Verification items for the finished model (mm, model axes). A direction names the side the tool comes from. Round coordinates to 2 decimals unless told otherwise and drop trailing zeros. Order: outer loops, then holes, each group sorted by start corner. A loop starts at its lowest first (then second) coordinate and runs counter-clockwise, first axis right, second up. Notation, with made-up numbers: M 84,73 L 130,73 A24 ccw 130,92 Z; hole C 27,73 d7. An arc over 180 degrees is marked long. Answer as a JSON object with one key per item and string values. Group by question number.
```python
from build123d import *

# Parameters (mm, degrees)
F_8_CLEARANCE_HOLE1_D     = 4.4958
F_8_CLEARANCE_HOLE1_DEPTH = 3.176
CIRPATTERN1_COUNT         = 6
SKETCH4_R                 = 63.5
CUT_EXTRUDE1_DEPTH        = 13.7


with BuildPart() as part:
    # Sketch1 → Revolve1 (revolve)
    with BuildSketch(Plane(origin=(0, 0, 0), x_dir=(0, 0, -1), z_dir=(1, 0, 0))):
        Polygon((66.675, 0), (69.85, 0), (69.85, 9.525), (82.55, 9.525), (82.55, 12.7), (0, 12.7), (0, 9.525), (66.675, 9.525), align=None)
    revolve(axis=Axis((0, 0, 0), (0, 1, 0)))

    # #8 Clearance Hole1
    with Locations(Plane(origin=(0, 12.7, 0), x_dir=(1, 0, 0), z_dir=(0, 1, 0))):
        with Locations((0, 76.2)):
            f_8_clearance_hole1 = Hole(F_8_CLEARANCE_HOLE1_D / 2, depth=F_8_CLEARANCE_HOLE1_DEPTH)

    # CirPattern1: #8 Clearance Hole1 ×6 about axis
    cirpattern1_axis = Axis((0, 0, 0), (0, 1, 0))
    for i in range(1, CIRPATTERN1_COUNT):
        add(f_8_clearance_hole1.rotate(cirpattern1_axis, i * 360 / CIRPATTERN1_COUNT), mode=Mode.SUBTRACT)

    # Sketch4 → Cut-Extrude1 (cut, through all)
    with BuildSketch(Plane(origin=(0, 12.7, 0), x_dir=(1, 0, 0), z_dir=(0, 1, 0))):
        Circle(SKETCH4_R)
    extrude(amount=-CUT_EXTRUDE1_DEPTH, mode=Mode.SUBTRACT)


solid = part.part
```
Q1. Cross-section at D-D, the plane x = -32. Record the cut outline in (y, z) (3 decimals).
Q2. Gauge pin test, flat ends, axial feed: pin 1 Ø7 at (x, z) = (0, 76.2) entering from -Y (3 decimals); pin 2 Ø4 at (x, y) = (-21, 10.5) entering from -Z; pin 3 Ø3.5 at (x, z) = (-65.99, 38.1) entering from +Y; pin 4 Ø1 at (y, z) = (9.5, -34) entering from -X. Record the tip position at first contact, or that the pin passes through.
Q3. Tool access check on faces 4 (the face through (26, 0, 62)), 5 (the face through (-20.027, 4.696, -63.596)). Record the directions out of +Z, -Z, +X, -X, +Y, -Y that give a thin tool (end or side, any length) a straight path to the whole face; none if there is none.
Q4. Cross-section at A-A, the plane z = 0. Record the cut outline in (x, y) (3 decimals).
Q5. Thickness scan on line 1 (Z direction, x = 0, y = 12); line 2 (X direction, y = 11.2, z = -38.1); line 3 (X direction, y = 11.6, z = 0). Record the ranges inside material, lowest first. Write a range as from..to.
Q6. Release check for a two-part mould opening along X. For faces 1 (the face through (42.503, 4.829, 55.431)), 2 (the face through (-0.29, 11.09, 78.43)), 3 (the face through (-19, 9.525, -68)) record: released by +X, released by -X, zero draft, split by the parting line, or undercut.
Q7. Cross-section at C-C, the plane z = 38.1. Record the cut outline in (x, y) (3 decimals), then the cut area to 3 significant figures.
Q8. Cross-section at B-B, the plane x = 0. Record the cut outline in (y, z) (3 decimals).
Conclusion:
{
 "1": {"outline": "M 0,-62.089 L 9.525,-62.089 L 9.525,-76.095 L 12.7,-76.095 L 12.7,-54.848 L 9.525,-54.848 L 9.525,-58.494 L 0,-58.494 Z; M 0,58.494 L 9.525,58.494 L 9.525,54.848 L 12.7,54.848 L 12.7,76.095 L 9.525,76.095 L 9.525,62.089 L 0,62.089 Z"},
 "2": {"pin 1": "y = 9.525", "pin 2": "z = -80.33", "pin 3": "through", "pin 4": "x = -75.45"},
 "3": {"face 4": "+Z, -Z, +X, -X, -Y", "face 5": "-Y"},
 "4": {"outline": "M -82.55,9.525 L -69.85,9.525 L -69.85,0 L -66.675,0 L -66.675,9.525 L -63.5,9.525 L -63.5,12.7 L -82.55,12.7 Z; M 63.5,9.525 L 66.675,9.525 L 66.675,0 L 69.85,0 L 69.85,9.525 L 82.55,9.525 L 82.55,12.7 L 63.5,12.7 Z"},
 "5": {"line 1": "-82.55..-78.45, -73.95..-63.5, 63.5..73.95, 78.45..82.55", "line 2": "-73.23..-68.24, -63.74..-50.8, 50.8..63.74, 68.24..73.23", "line 3": "-82.55..-63.5, 63.5..82.55"},
 "6": {"face 1": "split by the parting line", "face 2": "undercut", "face 3": "zero draft"},
 "7": {"outline": "M -73.232,9.525 L -68.239,9.525 L -68.239,12.7 L -73.232,12.7 Z; M -63.743,9.525 L -58.544,9.525 L -58.544,0 L -54.717,0 L -54.717,9.525 L -50.8,9.525 L -50.8,12.7 L -63.743,12.7 Z; M 50.8,9.525 L 54.717,9.525 L 54.717,0 L 58.544,0 L 58.544,9.525 L 63.743,9.525 L 63.743,12.7 L 50.8,12.7 Z; M 68.239,9.525 L 73.232,9.525 L 73.232,12.7 L 68.239,12.7 Z", "area": "187 mm2"},
 "8": {"outline": "M 0,-69.85 L 9.525,-69.85 L 9.525,-73.952 L 12.7,-73.952 L 12.7,-63.5 L 9.525,-63.5 L 9.525,-66.675 L 0,-66.675 Z; M 0,66.675 L 9.525,66.675 L 9.525,63.5 L 12.7,63.5 L 12.7,73.952 L 9.525,73.952 L 9.525,69.85 L 0,69.85 Z; M 9.525,-82.55 L 12.7,-82.55 L 12.7,-78.448 L 9.525,-78.448 Z; M 9.525,78.448 L 12.7,78.448 L 12.7,82.55 L 9.525,82.55 Z"}
}
